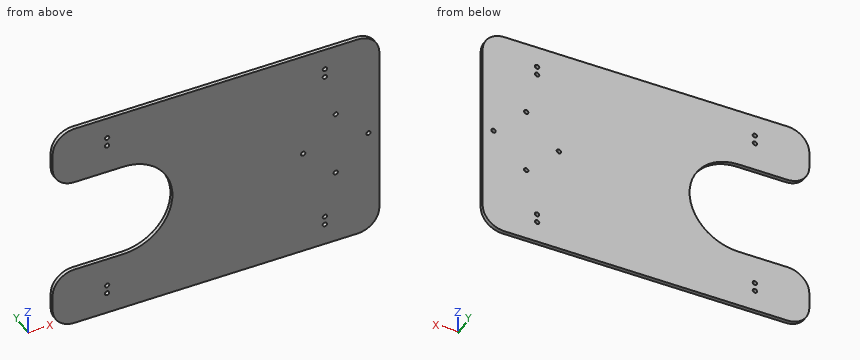
from build123d import *

# Parameters (mm, degrees)
SKETCH1_R           = 2
BOSS_EXTRUDE1_DEPTH = 1.75
FILLET1_R           = 20


with BuildPart() as part:
    # Sketch1 → Boss-Extrude1 (new, symmetric)
    with BuildSketch(Plane(origin=(0, 0, 0), x_dir=(1, 0, 0), z_dir=(0, 1, 0))):
        with BuildLine():
            Line((-150, 100), (-150, 45))
            Line((-150, 45), (-85, 45))
            ThreePointArc((-85, 45), (-40, 0), (-85, -45))
            Line((-85, -45), (-150, -45))
            Line((-150, -45), (-150, -100))
            Line((-150, -100), (150, -100))
            Line((150, -100), (150, 100))
            Line((150, 100), (-150, 100))
        make_face()
        with Locations(Location((-100, 80, 0), (0, 0, 270))):
            Circle(SKETCH1_R, mode=Mode.SUBTRACT)
        with Locations(Location((100, 80, 0), (0, 0, 270))):
            Circle(SKETCH1_R, mode=Mode.SUBTRACT)
        with Locations(Location((100, -80, 0), (0, 0, 270))):
            Circle(SKETCH1_R, mode=Mode.SUBTRACT)
        with Locations(Location((-100, -80, 0), (0, 0, 270))):
            Circle(SKETCH1_R, mode=Mode.SUBTRACT)
        with Locations(Location((-100, 72, 0), (0, 0, 270))):
            Circle(SKETCH1_R, mode=Mode.SUBTRACT)
        with Locations(Location((100, 72, 0), (0, 0, 270))):
            Circle(SKETCH1_R, mode=Mode.SUBTRACT)
        with Locations(Location((100, -72, 0), (0, 0, 270))):
            Circle(SKETCH1_R, mode=Mode.SUBTRACT)
        with Locations(Location((-100, -72, 0), (0, 0, 270))):
            Circle(SKETCH1_R, mode=Mode.SUBTRACT)
        with Locations(Location((110, 30, 0), (0, 0, 270))):
            Circle(SKETCH1_R, mode=Mode.SUBTRACT)
        with Locations(Location((140, 0, 0), (0, 0, 270))):
            Circle(SKETCH1_R, mode=Mode.SUBTRACT)
        with Locations(Location((110, -30, 0), (0, 0, 270))):
            Circle(SKETCH1_R, mode=Mode.SUBTRACT)
        with Locations(Location((80, 0, 0), (0, 0, 270))):
            Circle(SKETCH1_R, mode=Mode.SUBTRACT)
    extrude(amount=BOSS_EXTRUDE1_DEPTH, both=True)

    # Fillet1
    fillet1_edges = [part.edges().sort_by_distance(p)[0] for p in [
        (150, 0, 100),
        (-150, 0, 100),
        (-150, 0, 45),
        (-150, 0, -45),
        (-150, 0, -100),
        (150, 0, -100),
    ]]
    fillet(fillet1_edges, radius=FILLET1_R)


solid = part.part
Check sheet for the modelled part. Datum: model origin and axes. Units: mm. Give positions to 0.01 mm unless a question says otherwise; leave off trailing zeros. Loops run counter-clockwise (first coordinate to the right, second up) from the corner with the lowest first, then second, coordinate; pieces in that order, holes last. Notation, with made-up numbers: M 85,18 L 105,18 A22 cw 105,52 Z; hole C -15.5,-27.5 d10. An arc over 180 degrees is marked long. Return JSON: item names as keys, results as strings. Group by question number.
1. Cross-section at B-B on x = -91. Record the boundary of the cut face in (y, z), plus the area to 3 significant figures.
2. Thickness scan on L1, parallel to X at y = -0.45, z = -80; L2, parallel to X at y = -0.4, z = 0; L3, parallel to Z at x = -99, y = 1.6. Record the ranges inside material, lowest first.
3. Cross-section at A-A on y = -0.2. State how many separate pieces and enclosed holes the cut face has, plus the area to 3 significant figures.
Return value:
{
 "1": {"outline": "M -1.75,-100 L 1.75,-100 L 1.75,-45 L -1.75,-45 Z; M -1.75,45 L 1.75,45 L 1.75,100 L -1.75,100 Z", "area": "385 mm^2"},
 "2": {"L1": "-150 to -102, -98 to 98, 102 to 150", "L2": "-40 to 78, 82 to 138, 142 to 150", "L3": "-100 to -81.73, -78.27 to -73.73, -70.27 to -45, 45 to 70.27, 73.73 to 78.27, 81.73 to 100"},
 "3": {"separate pieces": "1", "enclosed holes": "12", "area": "50,300 mm^2"}
}
